CAD build for the part. Positions are in the model's coordinates, mm. A direction names the side the tool comes from. Round coordinates to 2 decimals unless told otherwise and drop trailing zeros. Order: outer loops, then holes, each group sorted by start corner. A loop starts at its lowest first (then second) coordinate and runs counter-clockwise, first axis right, second up. Notation, with made-up numbers: M 43.25,-35.75 L 66.25,-35.75 A18 cw 66.25,-7.75 Z; hole C 68.5,-40 d8. An arc over 180 degrees is marked long. Answer as a JSON object with one key per item and string values.
```python
from build123d import *

# Parameters (mm, degrees)
F0_R          = 4.75
F1_DEPTH      = 10
F1_DEPTH_BACK = 5
F0_W          = 120
F0_H          = 18
F2_DEPTH      = 5


with BuildPart() as f1:
    # F0 (on Front) → F1 (new body, two sides)
    with BuildSketch(Plane.XZ) as f1_sk:
        Circle(F0_R)
    extrude(amount=F1_DEPTH)
    extrude(f1_sk.sketch, amount=-F1_DEPTH_BACK)



with BuildPart() as f1b:
    # F0 (on Front) → F1, piece 2 (new body, two sides)
    with BuildSketch(Plane.XZ) as f1_2_sk:
        with Locations((95, 0)):
            Circle(F0_R)
    extrude(amount=F1_DEPTH)
    extrude(f1_2_sk.sketch, amount=-F1_DEPTH_BACK)


with BuildPart() as f1_1:
    add(f1.part)

    add(f1b.part)  # F2 merges F1b
    # F0 (on Front) → F2 (join)
    with BuildSketch(Plane.XZ):
        with Locations((47.7674523741, 0.1763370037)):
            Rectangle(F0_W, F0_H)
        Circle(F0_R, mode=Mode.SUBTRACT)
        with Locations((95, 0)):
            Circle(F0_R, mode=Mode.SUBTRACT)
    extrude(amount=-F2_DEPTH)


solid = f1_1.part
```
Item 1: Drop flat-ended pins along their axis: pin 1 Ø3 at (x, y) = (4.5, -1) entering from +Z; pin 2 Ø2 at (y, z) = (-2.5, -1.5) entering from +X. Give the stop position or say it passes through.
Worked answers:
{"pin 1": "stops at z = 9.18", "pin 2": "stops at x = 99.72"}
Item 2: Saw through at A-A on z = 0. List the corners of the cut face in (x, y).
Worked answers:
{"outline": "M -12.23,0 L -4.75,0 L -4.75,-10 L 4.75,-10 L 4.75,0 L 90.25,0 L 90.25,-10 L 99.75,-10 L 99.75,0 L 107.77,0 L 107.77,5 L -12.23,5 Z"}
Item 3: Saw through at C-C on y = -4.75. List the corners of the cut face in (x, z), and give its area (3 significant figures).
Worked answers:
{"outline": "C 0,0 d9.5; C 95,0 d9.5", "area": "142 mm2"}
Item 4: Wall check: line 1 along Y through (x, z) = (60, -1.5); line 2 along X through (y, z) = (-1.75, -4.25); line 3 along X through (y, z) = (-8.25, 3). Give the ranges that are in metal, low to high. Write a range as [from, to].
Worked answers:
{"line 1": "y = [0, 5]", "line 2": "x = [-2.12, 2.12], [92.88, 97.12]", "line 3": "x = [-3.68, 3.68], [91.32, 98.68]"}
Item 5: Saw through at D-D on z = -6. List the corners of the cut face in (x, y), and give its area (3 significant figures).
Worked answers:
{"outline": "M -12.23,0 L 107.77,0 L 107.77,5 L -12.23,5 Z", "area": "600 mm2"}
Item 6: Two-plate mould, pull along X, no slides. Class faces 3 (the flat face through (0, -10, 0)), 4 (the flat face through (-12.233, 2, 0)), 5 (the cylindrical face through (99.53, -5.07, 1.43)), 6 (the flat face through (107.767, 2, 0)): released by +X, released by -X, zero draft, split by the parting line, or undercut.
Worked answers:
{"face 3": "zero draft", "face 4": "released by -X", "face 5": "undercut", "face 6": "released by +X"}
Item 7: 3-axis set-ups, long thin cutter, end or side, ignore diameter. For faces 1 (the cylindrical face through (2.192, -5.07, -4.214)), 2 (the flat face through (47, 2, -8.824)): which of +Z, -Z, +X, -X, +Y, -Y reach the whole face in a straight line?
Worked answers:
{"face 1": "-Y", "face 2": "-Z, +X, -X, +Y, -Y"}
Item 8: Saw through at B-B on x = 95. List the corners of the cut face in (y, z).
Worked answers:
{"outline": "M -10,-4.75 L 0,-4.75 L 0,-8.82 L 5,-8.82 L 5,9.18 L 0,9.18 L 0,4.75 L -10,4.75 Z"}
